```python
from build123d import *

# Parameters (mm, degrees)
SKETCH1_R           = 2.6
BOSS_EXTRUDE1_DEPTH = 4
FILLET1_R           = 5


with BuildPart() as part:
    # Sketch1 → Boss-Extrude1 (new body)
    with BuildSketch(Plane.XY):
        Polygon((-17, -51.749074061), (17, -51.749074061), (42, -18), (42, 18), (-42, 18), (-42, -18), align=None)
        with Locations((-15.5, 10.75)):
            Circle(SKETCH1_R, mode=Mode.SUBTRACT)
        with Locations((15.5, 10.75)):
            Circle(SKETCH1_R, mode=Mode.SUBTRACT)
        with Locations((-26.75, -18)):
            Circle(SKETCH1_R, mode=Mode.SUBTRACT)
        with Locations((26.75, -18)):
            Circle(SKETCH1_R, mode=Mode.SUBTRACT)
        with Locations((-11.5, -44.499074061)):
            Circle(SKETCH1_R, mode=Mode.SUBTRACT)
        with Locations((11.5, -44.499074061)):
            Circle(SKETCH1_R, mode=Mode.SUBTRACT)
    extrude(amount=BOSS_EXTRUDE1_DEPTH)

    # Fillet1
    fillet1_edges = [part.edges().sort_by_distance(p)[0] for p in [
        (17, -51.749074061, 2),
        (-17, -51.749074061, 2),
        (-42, -18, 2),
        (-42, 18, 2),
        (42, 18, 2),
        (42, -18, 2),
    ]]
    fillet(fillet1_edges, radius=FILLET1_R)


solid = part.part
```
Could you check a few things on this model? Use its own coordinates, in mm. Give positions to 0.01 mm unless a question says otherwise; leave off trailing zeros. Order: outer loops, then holes, each group sorted by start corner. A loop starts at its lowest first (then second) coordinate and runs counter-clockwise, first axis right, second up.
Q1. If I drill on line 1 along Y through (x, z) = (11.5, 2.8); line 2 along Y through (x, z) = (26, 3); line 3 along X through (y, z) = (-18.5, 3.5), over which ranges is the centre line in solid material (lowest first)?
Q2. Suppose I cut it at B-B, the plane x = 26.75. Write out the boundary of the cut face in (y, z).
Q3. Suppose I cut it at C-C, the plane z = 1.7. Write out the boundary of the cut face in (x, y).
Q4. Suppose I cut it at D-D, the plane x = -11.5. Write out the boundary of the cut face in (y, z), and give its area (3 significant figures).
Q5. Suppose I cut it at A-A, the plane y = 10.75. Write out the boundary of the cut face in (x, z).
Q6. We'd pull the mould along X, two halves only. Please class faces 1 (the cylindrical face through (-13.1, 9.75, 1.97)), 2 (the flat face through (-42, -1, 2)), 3 (the flat face through (29.6, -34.74, 1.97)), 4 (the flat face through (-1, -16, 0)): +X half, -X half, draft (parallel to the pull), parting line (faces both ways), or undercut.
Solution:
1. line 1: y = -51.75 to -47.1, -41.9 to 18
1. line 2: y = -39.6 to -20.49, -15.51 to 18
1. line 3: x = -41.51 to -29.3, -24.2 to 24.2, 29.3 to 41.51
2. outline: (-38.59, 0) - (-20.6, 0) - (-20.6, 4) - (-38.59, 4) - close; (-15.4, 0) - (18, 0) - (18, 4) - (-15.4, 4) - close
3. outline: (-42, -16.35) arc R5 ccw to (-41.02, -19.33) - (-18.5, -49.73) arc R5 ccw to (-14.48, -51.75) - (14.48, -51.75) arc R5 ccw to (18.5, -49.73) - (41.02, -19.33) arc R5 ccw to (42, -16.35) - (42, 13) arc R5 ccw to (37, 18) - (-37, 18) arc R5 ccw to (-42, 13) - close; hole circle Ø5.2 at (-26.75, -18); hole circle Ø5.2 at (-15.5, 10.75); hole circle Ø5.2 at (-11.5, -44.5); hole circle Ø5.2 at (11.5, -44.5); hole circle Ø5.2 at (15.5, 10.75); hole circle Ø5.2 at (26.75, -18)
4. outline: (-51.75, 0) - (-47.1, 0) - (-47.1, 4) - (-51.75, 4) - close; (-41.9, 0) - (18, 0) - (18, 4) - (-41.9, 4) - close
4. area: 258 mm2
5. outline: (-42, 0) - (-18.1, 0) - (-18.1, 4) - (-42, 4) - close; (-12.9, 0) - (12.9, 0) - (12.9, 4) - (-12.9, 4) - close; (18.1, 0) - (42, 0) - (42, 4) - (18.1, 4) - close
6. face 1: undercut
6. face 2: -X half
6. face 3: +X half
6. face 4: draft
